from build123d import *

# Parameters (mm, degrees)
BOSS_EXTRUDE1_DEPTH = 20.32
CUT_EXTRUDE1_DEPTH  = 12.7
SKETCH14_R          = 8.0645
CUT_EXTRUDE4_DEPTH  = 16.002
CUT_EXTRUDE5_DEPTH  = 34.544
SKETCH14_5_R        = 3.048
CUT_EXTRUDE6_DEPTH  = 157.413445344
SKETCH15_W          = 35.898582
SKETCH15_H          = 38.980588406
CUT_EXTRUDE7_DEPTH  = 17.78
SKETCH16_W          = 41.91
SKETCH16_H          = 2.54
BOSS_EXTRUDE2_DEPTH = 12.7
CUT_EXTRUDE9_DEPTH  = 11.4
SKETCH17_5_R        = 10
CUT_EXTRUDE10_DEPTH = 11.4
CUT_EXTRUDE16_DEPTH = 10
SKETCH25_W          = 35.898582
SKETCH25_H          = 38.980588406
BOSS_EXTRUDE4_DEPTH = 5.08


with BuildPart() as part:
    # Sketch3 → Boss-Extrude1 (new body)
    with BuildSketch(Plane(origin=(0, 0, 0), x_dir=(1, 0, 0), z_dir=(0, 1, 0))):
        with BuildLine():
            Line((101.599873, 0), (110.066582, 0))
            Line((110.066582, 0), (110.066582, 42.333418))
            Line((110.066582, 42.333418), (55.033291, 42.333418))
            Line((55.033291, 42.333418), (8.4666328, 42.333418))
            Line((8.4666328, 42.333418), (0, 42.333418))
            Line((0, 42.333418), (0, 0))
            Line((0, 0), (8.4666328, 0))
            Line((8.4666328, 0), (8.4666328, -25.4))
            Line((8.4666328, -25.4), (12.6999492, -35.56))
            Line((12.6999492, -35.56), (12.6999492, -69.426582))
            add(Edge.make_bspline(
                [(12.6999492, -69.426582), (11.690404189, -80.766544706), (8.46666328, -91.44)],
                knots=[0, 0, 0, 0.504540069, 0.504540069, 0.504540069], degree=2))
            Line((8.46666328, -91.44), (8.46666328, -111.76))
            Line((8.46666328, -111.76), (101.599995682, -111.76))
            Line((101.599995682, -111.76), (101.599995682, -91.44))
            add(Edge.make_bspline(
                [(97.366709, -69.426582), (98.376270675, -80.766537876), (101.599995682, -91.44)],
                knots=[0, 0, 0, 0.504540407, 0.504540407, 0.504540407], degree=2))
            Line((97.366709, -69.426582), (97.366709, -35.56))
            Line((97.366709, -35.56), (101.599873, -25.4))
            Line((101.599873, -25.4), (101.599873, 0))
        make_face()
    extrude(amount=BOSS_EXTRUDE1_DEPTH)

    # Sketch7 → Cut-Extrude1 (cut)
    with BuildSketch(Plane(origin=(0, 20.32, 0), x_dir=(1, 0, 0), z_dir=(0, 1, 0))):
        with BuildLine():
            Line((16.0866328, 0), (93.979873, 0))
            Line((93.979873, 0), (93.979873, -23.876056271))
            Line((93.979873, -23.876056271), (89.746709, -34.036056271))
            Line((89.746709, -34.036056271), (89.746709, -69.759644388))
            add(Edge.make_bspline(
                [(89.746709, -69.759644388), (90.418698914, -77.556217584), (91.829471112, -85.161374913), (93.979995682, -92.545959033)],
                knots=[0, 0, 0, 0, 1, 1, 1, 1], degree=3))
            Line((93.979995682, -92.545959033), (93.979995682, -104.14))
            Line((93.979995682, -104.14), (16.08666328, -104.14))
            Line((16.08666328, -104.14), (16.08666328, -92.545964634))
            add(Edge.make_bspline(
                [(16.08666328, -92.545964634), (18.237198531, -85.161380775), (19.647970427, -77.556219246), (20.3199492, -69.759638641)],
                knots=[0, 0, 0, 0, 1, 1, 1, 1], degree=3))
            Line((20.3199492, -69.759638641), (20.3199492, -34.036005627))
            Line((20.3199492, -34.036005627), (16.0866328, -23.876005627))
            Line((16.0866328, -23.876005627), (16.0866328, 0))
        make_face()
    extrude(amount=-CUT_EXTRUDE1_DEPTH, mode=Mode.SUBTRACT)

    # Sketch14 → Cut-Extrude4 (cut)
    with BuildSketch(Plane.ZY.offset(-2.54)):
        with Locations((-21.166709, 20.32)):
            Circle(SKETCH14_R)
    cut_extrude4 = extrude(amount=-CUT_EXTRUDE4_DEPTH, mode=Mode.SUBTRACT)

    # Sketch14<4> → Cut-Extrude5 (cut)
    with BuildSketch(Plane.ZY.offset(-2.54)):
        with BuildLine():
            Line((-26.672257875, 14.4272), (-15.661160125, 14.4272))
            ThreePointArc((-15.661160125, 14.4272), (-21.166709, 28.3845), (-26.672257875, 14.4272))
        make_face()
    cut_extrude5 = extrude(amount=-CUT_EXTRUDE5_DEPTH, mode=Mode.SUBTRACT)

    # Sketch14<5> → Cut-Extrude6 (cut, through all)
    with BuildSketch(Plane.ZY.offset(-2.54)):
        with Locations((-21.166709, 20.32)):
            Circle(SKETCH14_5_R)
    cut_extrude6 = extrude(amount=CUT_EXTRUDE6_DEPTH, mode=Mode.SUBTRACT)

    # Mirror2: Cut-Extrude4, Cut-Extrude5, Cut-Extrude6 across plane
    add(cut_extrude4.mirror(Plane(origin=(55.033291, 0, 0), x_dir=(0, 0, 1), z_dir=(1, 0, 0))), mode=Mode.SUBTRACT)
    add(cut_extrude5.mirror(Plane(origin=(55.033291, 0, 0), x_dir=(0, 0, 1), z_dir=(1, 0, 0))), mode=Mode.SUBTRACT)
    add(cut_extrude6.mirror(Plane(origin=(55.033291, 0, 0), x_dir=(0, 0, 1), z_dir=(1, 0, 0))), mode=Mode.SUBTRACT)

    # Sketch15 → Cut-Extrude7 (cut)
    with BuildSketch(Plane(origin=(0, 20.32, 0), x_dir=(1, 0, 0), z_dir=(0, 1, 0))):
        with Locations((55.033291, 19.490294203)):
            Rectangle(SKETCH15_W, SKETCH15_H)
    extrude(amount=-CUT_EXTRUDE7_DEPTH, mode=Mode.SUBTRACT)

    # Sketch16 → Boss-Extrude2 (add)
    with BuildSketch(Plane(origin=(0, 7.62, 0), x_dir=(1, 0, 0), z_dir=(0, 1, 0))):
        with Locations((55.0333291, -15.57585033)):
            Rectangle(SKETCH16_W, SKETCH16_H)
        Polygon((75.9883291, -21.92585033), (73.4483291, -21.92585033), (73.4483291, -86.94985033), (36.6183291, -86.94985033), (36.6183291, -21.92585033), (34.0783291, -21.92585033), (34.0783291, -89.48985033), (75.9883291, -89.48985033), align=None)
    extrude(amount=BOSS_EXTRUDE2_DEPTH)

    # Sketch17 → Cut-Extrude9 (cut)
    with BuildSketch(Plane(origin=(104.139873, 0, 0), x_dir=(0, 0, -1), z_dir=(1, 0, 0))):
        with BuildLine():
            Line((-13.75, 9.42), (-12.7, 9.42))
            Line((-12.7, 9.42), (-11.65, 9.42))
            Line((-11.65, 9.42), (-11.65, 10.375277782))
            ThreePointArc((-11.65, 10.375277782), (-12.7, 10.32), (-13.75, 10.375277782))
            Line((-13.75, 10.375277782), (-13.75, 9.42))
        make_face()
    extrude(amount=-CUT_EXTRUDE9_DEPTH, mode=Mode.SUBTRACT)

    # Sketch17<5> → Cut-Extrude10 (cut)
    with BuildSketch(Plane(origin=(104.139873, 0, 0), x_dir=(0, 0, -1), z_dir=(1, 0, 0))):
        with Locations((-12.7, 20.32)):
            Circle(SKETCH17_5_R)
    extrude(amount=-CUT_EXTRUDE10_DEPTH, mode=Mode.SUBTRACT)

    # Sketch23 → Cut-Extrude16 (cut)
    with BuildSketch(Plane.XY.offset(-38.980588406)):
        Polygon((62.653291, 14.986), (62.653291, 7.62), (55.033291, 7.62), (47.413291, 7.62), (47.413291, 14.986), align=None)
    extrude(amount=-CUT_EXTRUDE16_DEPTH, mode=Mode.SUBTRACT)

    # Sketch25 → Boss-Extrude4 (add)
    with BuildSketch(Plane(origin=(0, 2.54, 0), x_dir=(1, 0, 0), z_dir=(0, 1, 0))):
        with Locations((55.033291, 19.490294203)):
            Rectangle(SKETCH25_W, SKETCH25_H)
    extrude(amount=BOSS_EXTRUDE4_DEPTH)


solid = part.part
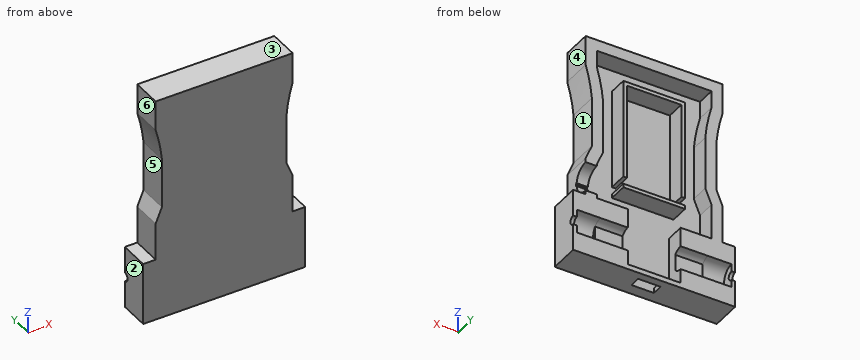
Build history of the part. All positions in model axes, mm. Face numbers are marked on the shaded views. A direction names the side the tool comes from. Coordinates: 2 decimals unless noted, no trailing zeros. Order: outer loops, then holes, each group sorted by start corner. A loop starts at its lowest first (then second) coordinate and runs counter-clockwise, first axis right, second up. Notation, with made-up numbers: (-9.75, 79) - (2.25, 79) arc R26 ccw to (2.25, 110) - close; hole circle Ø9 at (27.5, -27). An arc over 180 degrees is marked (long way). Write item = value, one per line. Start each with the question number.
1) 3-axis set-ups, long thin cutter, end or side, ignore diameter. For the marked faces 4, 5 and 6: which of +Z, -Z, +X, -X, +Y, -Y reach the whole face in a straight line?
2) Saw through at B-B on x = 45. Write the cut outline in (y, z).
3) Saw through at C-C on z = 42. Write the cut outline in (x, y).
4) Saw through at A-A on z = 95. Write the cut outline in (x, y).
5) Wall check: line 1 along X through (y, z) = (19.5, 69); line 2 along Z through (x, y) = (37, 9.5); line 3 along Z through (x, y) = (39.5, 16.25). Give the ranges that are in metal, low to high. Write a range as from..to.
6) Two-plate mould, pull along Z, no slides. Class the marked faces 1, 2 and 3: pulls with the +Z half, pulls with the -Z half, needs draft (parallel to the pull), parting line crosses it, or undercut.
7) Saw through at D-D on x = 80. Write the cut outline in (y, z).
8) Flat gauge pins, fed straight in: pin 1 Ø10 at (y, z) = (12, 8) entering from +X; pin 2 Ø12 at (y, z) = (14, 15) entering from -X; pin 3 Ø6.5 at (y, z) = (11.5, 52) entering from -X. Where does each tip first touch, or does it go through?
From the geometry:
q1.face_4 = +Z, +X, +Y, -Y
q1.face_5 = -X, +Y, -Y
q1.face_6 = +Z, -X, +Y, -Y
q2.outline = (0, -42.33) - (20.32, -42.33) - (20.32, -38.98) - (7.62, -38.98) - (7.62, 14.31) - (20.32, 14.31) - (20.32, 16.85) - (7.62, 16.85) - (7.62, 86.95) - (20.32, 86.95) - (20.32, 89.49) - (7.62, 89.49) - (7.62, 104.14) - (20.32, 104.14) - (20.32, 111.76) - (0, 111.76) - close
q3.outline = (12.7, 0) - (97.37, 0) - (97.37, 20.32) - (89.75, 20.32) - (89.75, 7.62) - (75.99, 7.62) - (75.99, 20.32) - (73.45, 20.32) - (73.45, 7.62) - (36.62, 7.62) - (36.62, 20.32) - (34.08, 20.32) - (34.08, 7.62) - (20.32, 7.62) - (20.32, 20.32) - (12.7, 20.32) - close
q4.outline = (8.47, 0) - (101.6, 0) - (101.6, 20.32) - (93.98, 20.32) - (93.98, 7.62) - (16.09, 7.62) - (16.09, 20.32) - (8.47, 20.32) - close
q5.line_1 = 12.7..20.32, 34.08..36.62, 73.45..75.99, 89.75..97.37
q5.line_2 = -42.33..0, 14.31..16.85, 86.95..89.49, 104.14..111.76
q5.line_3 = -42.33..-38.98, 14.31..16.85, 86.95..89.49, 104.14..111.76
q6.face_1 = undercut
q6.face_2 = needs draft
q6.face_3 = pulls with the +Z half
q7.outline = (0, -42.33) - (20.32, -42.33) - (20.32, -29.23) arc R8.06 cw to (14.43, -26.67) - (14.43, -15.66) arc R8.06 cw to (20.32, -13.1) - (20.32, 0) - (7.62, 0) - (7.62, 104.14) - (20.32, 104.14) - (20.32, 111.76) - (0, 111.76) - close
q8.pin_1 = 101.6
q8.pin_2 = 8.47
q8.pin_3 = 12.7
